Source: CAD feature listing. Evaluate the final solid. Frame: model axes, mm. A direction names the side the tool comes from. Give positions to 0.01 mm unless a question says otherwise; leave off trailing zeros. Loops run counter-clockwise (first coordinate to the right, second up) from the corner with the lowest first, then second, coordinate; pieces in that order, holes last. Notation, with made-up numbers: M -10,46 L 0,46 A5 cw 0,55 Z; hole C 55,44.25 d2. An arc over 180 degrees is marked long. Write item = value, one per line.
from build123d import *

# Parameters (mm, degrees)
BOSS_EXTRUDE1_DEPTH             = 3.175
F_10_CLEARANCE_HOLE1_AT_2_COUNT = 2
F_10_CLEARANCE_HOLE1_AT_2_PITCH = 19.05
F_10_CLEARANCE_HOLE1_AT_3_COUNT = 2
F_10_CLEARANCE_HOLE1_AT_3_PITCH = 44.45
F_10_CLEARANCE_HOLE1_AT_4_COUNT = 2
F_10_CLEARANCE_HOLE1_AT_4_PITCH = 25.4
F_10_CLEARANCE_HOLE1_AT_5_COUNT = 2
F_10_CLEARANCE_HOLE1_AT_5_PITCH = 50.8


with BuildPart() as part:
    # Sketch1 → Boss-Extrude1 (new body)
    with BuildSketch(Plane.XY):
        Polygon((-260.753367516, 0), (-273.453367516, 0), (-273.453367516, 63.5), (-260.753367516, 63.5), (-260.753367516, 25.4), (-248.053367516, 12.7), (-203.603367516, 12.7), (-203.603367516, 0), align=None)
    extrude(amount=BOSS_EXTRUDE1_DEPTH)

    # Sketch4 → #10 Clearance Hole1 (revolve, cut)
    with BuildSketch(Plane(origin=(-267.103367516, 6.35, 3.175), x_dir=(0, -1, 0), z_dir=(1, 0, 0))):
        Polygon((0, 0), (0, 3.175), (2.4892, 3.175), (2.4892, 3.141080936), (5.2197, 0), align=None)
    f_10_clearance_hole1 = revolve(axis=Axis((-267.103367516, 6.35, 9.525), (0, 0, -1)), mode=Mode.SUBTRACT)

    # #10 Clearance Hole1 at 2: #10 Clearance Hole1 ×2
    with Locations(*[(0, i * F_10_CLEARANCE_HOLE1_AT_2_PITCH, 0) for i in range(1, F_10_CLEARANCE_HOLE1_AT_2_COUNT)]):
        add(f_10_clearance_hole1, mode=Mode.SUBTRACT)

    # #10 Clearance Hole1 at 3: #10 Clearance Hole1 ×2
    with Locations(*[(0, i * F_10_CLEARANCE_HOLE1_AT_3_PITCH, 0) for i in range(1, F_10_CLEARANCE_HOLE1_AT_3_COUNT)]):
        add(f_10_clearance_hole1, mode=Mode.SUBTRACT)

    # #10 Clearance Hole1 at 4: #10 Clearance Hole1 ×2
    with Locations(*[(i * F_10_CLEARANCE_HOLE1_AT_4_PITCH, 0, 0) for i in range(1, F_10_CLEARANCE_HOLE1_AT_4_COUNT)]):
        add(f_10_clearance_hole1, mode=Mode.SUBTRACT)

    # #10 Clearance Hole1 at 5: #10 Clearance Hole1 ×2
    with Locations(*[(i * F_10_CLEARANCE_HOLE1_AT_5_PITCH, 0, 0) for i in range(1, F_10_CLEARANCE_HOLE1_AT_5_COUNT)]):
        add(f_10_clearance_hole1, mode=Mode.SUBTRACT)


solid = part.part
1. Cut plane D-D, the plane x = -232. Return the cut outline in (y, z) (3 decimals).
Derived:
outline = M 0,0 L 12.7,0 L 12.7,3.175 L 0,3.175 Z
2. Reachability of faces 1 (the flat face through (-273.453, 31, 2)), 2 (the flat face through (-226, 12.7, 2)) from +Z, -Z, +X, -X, +Y, -Y: full face, straight path, thin tool, end or side. Return the list, or none.
Derived:
face_1 = +Z, -Z, -X, +Y, -Y
face_2 = +Z, -Z, +X, +Y
3. Cut plane C-C, the plane z = 2.1. Return the cut outline in (x, y), then the cut area to 3 significant figures.
Derived:
outline = M -273.45,0 L -203.6,0 L -203.6,12.7 L -248.05,12.7 L -260.75,25.4 L -260.75,63.5 L -273.45,63.5 Z; hole C -267.1,6.35 d8.57; hole C -267.1,25.4 d8.57; hole C -267.1,50.8 d8.57; hole C -241.7,6.35 d8.57; hole C -216.3,6.35 d8.57
area = 1,320 mm²
4. Cut plane A-A, the plane y = 6.35. Return the cut outline in (x, z) (3 decimals), then the cut area to 3 significant figures.
Derived:
outline = M -273.453,0 L -269.593,0 L -269.593,0.034 L -272.323,3.175 L -273.453,3.175 Z; M -264.614,0 L -244.193,0 L -244.193,0.034 L -246.923,3.175 L -261.884,3.175 L -264.614,0.034 Z; M -239.214,0 L -218.793,0 L -218.793,0.034 L -221.523,3.175 L -236.484,3.175 L -239.214,0.034 Z; M -213.814,0 L -203.603,0 L -203.603,3.175 L -211.084,3.175 L -213.814,0.034 Z
area = 149 mm²
5. Cut plane B-B, the plane y = 50.8. Return the cut outline in (x, z) (3 decimals), then the cut area to 3 significant figures.
Derived:
outline = M -273.453,0 L -269.593,0 L -269.593,0.034 L -272.323,3.175 L -273.453,3.175 Z; M -264.614,0 L -260.753,0 L -260.753,3.175 L -261.884,3.175 L -264.614,0.034 Z
area = 15.9 mm²
6. First-contact query: pin 1 Ø1.6 at (y, z) = (52, 1) entering from +X. Flat tip, straight axial feed; report the tip coordinate or a pass-through.
Derived:
pin_1 = -260.75
7. Pull-direction query (X, two-part tool) for faces 3 (the flat face through (-260.753, 45, 2)), 4 (the flat face through (-239, 0, 2)), 5 (the conical face through (-243.9, 4.9, 0.2)); classes: +X half, -X half, draft (parallel to the pull), parting line (faces both ways), or undercut.
Derived:
face_3 = +X half
face_4 = draft
face_5 = undercut
8. Material intervals for probe 1 along X at (y, z) = (6.35, 0.05); probe 2 along X at (y, z) = (50.8, 0.05); probe 3 along Y at (x, z) = (-231, 1.95), sorted ascending. Write a range as from..to.
Derived:
probe_1 = -273.45..-269.61, -264.6..-244.21, -239.2..-218.81, -213.8..-203.6
probe_2 = -273.45..-269.61, -264.6..-260.75
probe_3 = 0..12.7
